from build123d import *

# Parameters (mm, degrees)
SKETCH1_W           = 73.66
SKETCH1_H           = 127
BOSS_EXTRUDE1_DEPTH = 3.175
SKETCH2_W           = 25.4
SKETCH2_H           = 3.175
BOSS_EXTRUDE2_DEPTH = 3.175
SKETCH3_W           = 25.4
SKETCH3_H           = 3.175
BOSS_EXTRUDE3_DEPTH = 3.175
SKETCH5_W           = 25.4
SKETCH5_H           = 3.175
BOSS_EXTRUDE4_DEPTH = 3.175


with BuildPart() as part:
    # Sketch1 → Boss-Extrude1 (new body)
    with BuildSketch(Plane(origin=(0, 0, 0), x_dir=(1, 0, 0), z_dir=(0, 1, 0))):
        with Locations((38.311666667, 4.7625)):
            Rectangle(SKETCH1_W, SKETCH1_H)
    extrude(amount=BOSS_EXTRUDE1_DEPTH)

    # Sketch2 → Boss-Extrude2 (add)
    with BuildSketch(Plane(origin=(75.141666667, 0, 0), x_dir=(0, 0, -1), z_dir=(1, 0, 0))):
        with Locations((4.7625, 1.5875)):
            Rectangle(SKETCH2_W, SKETCH2_H)
    extrude(amount=BOSS_EXTRUDE2_DEPTH)

    # Sketch3 → Boss-Extrude3 (add)
    with BuildSketch(Plane.XY.offset(58.7375)):
        with Locations((27.389666667, 1.5875)):
            Rectangle(SKETCH3_W, SKETCH3_H)
    extrude(amount=BOSS_EXTRUDE3_DEPTH)

    # Sketch5 → Boss-Extrude4 (add)
    with BuildSketch(Plane(origin=(0, 0, -68.2625), x_dir=(-1, 0, 0), z_dir=(0, 0, -1))):
        with Locations((-27.389666667, 1.5875)):
            Rectangle(SKETCH5_W, SKETCH5_H)
    extrude(amount=BOSS_EXTRUDE4_DEPTH)


solid = part.part
Design review of the part built by this model. Coordinates are the model's own, in mm. A direction names the side the tool comes from. Round coordinates to 2 decimals unless told otherwise and drop trailing zeros. Order: outer loops, then holes, each group sorted by start corner. A loop starts at its lowest first (then second) coordinate and runs counter-clockwise, first axis right, second up.
1) Machinability: for faces 1 (the flat face through (77, 2, -17.462)), 2 (the flat face through (77, 2, 7.937)), 3 (the flat face through (8, 2, 58.738)), which of the approach directions +Z, -Z, +X, -X, +Y, -Y give a long, thin tool a straight path to every point of the face, cutting with its end or side? Answer none if there is none.
The answers:
face 1: -Z, +X, +Y, -Y
face 2: +Z, +X, +Y, -Y
face 3: +Z, -X, +Y, -Y
2) Consider section B-B (x = 51). State the section outline as (y, z) points (1 decimal), plus the area to 3 significant figures.
The answers:
outline: (0, -68.3) - (3.2, -68.3) - (3.2, 58.7) - (0, 58.7) - close
area: 403 mm2
3) Consider section C-C (z = 14). State the section outline as (x, y) points (3 decimals), plus the area to 3 significant figures.
The answers:
outline: (1.482, 0) - (75.142, 0) - (75.142, 3.175) - (1.482, 3.175) - close
area: 234 mm2
4) For L1, parallel to X at y = 0.7, z = -33; L2, parallel to Z at x = 8, y = 0.65, list the stretches that pass through material, from the lowest coordinate up.
The answers:
L1: x = 1.48 to 75.14
L2: z = -68.26 to 58.74
5) Consider section A-A (y = 2.3). State the section outline as (x, z) points.
The answers:
outline: (1.48, -68.26) - (14.69, -68.26) - (14.69, -71.44) - (40.09, -71.44) - (40.09, -68.26) - (75.14, -68.26) - (75.14, -17.46) - (78.32, -17.46) - (78.32, 7.94) - (75.14, 7.94) - (75.14, 58.74) - (40.09, 58.74) - (40.09, 61.91) - (14.69, 61.91) - (14.69, 58.74) - (1.48, 58.74) - close
6) Clearance check with flat-ended pins moving along their axes: pin 1 Ø1 at (y, z) = (1.5, 60) entering from +X; pin 2 Ø1 at (y, z) = (2, 22) entering from +X; pin 3 Ø1 at (x, y) = (76.5, 1.5) entering from -Z. State where each tip first meets the part, or that it passes through.
The answers:
pin 1: stops at x = 40.09
pin 2: stops at x = 75.14
pin 3: stops at z = -17.46
